from build123d import *

# Parameters (mm, degrees)
SKETCH1_W           = 669.925
SKETCH1_H           = 95.73895
BOSS_EXTRUDE1_DEPTH = 19.05
SKETCH2_R           = 12.7
CUT_EXTRUDE4_DEPTH  = 20.05


with BuildPart() as part:
    # Sketch1 → Boss-Extrude1 (new body)
    with BuildSketch(Plane(origin=(0, 0, 0), x_dir=(1, 0, 0), z_dir=(0, 1, 0))):
        with Locations((334.9625, 47.869475)):
            Rectangle(SKETCH1_W, SKETCH1_H)
    extrude(amount=BOSS_EXTRUDE1_DEPTH)

    # Sketch2 → Cut-Extrude4 (cut, through all)
    with BuildSketch(Plane.XZ):
        with Locations((334.9625, -82.78495)):
            Circle(SKETCH2_R)
    extrude(amount=-CUT_EXTRUDE4_DEPTH, mode=Mode.SUBTRACT)


solid = part.part
The listing builds one solid part. Answer for the finished solid, in the listing's coordinates (mm). Give positions to 0.01 mm unless a question says otherwise; leave off trailing zeros. Write each loop counter-clockwise with the first axis right and the second up, starting at its lowest first coordinate (ties: lowest second). Pieces come first, ordered by that corner, then holes.
1) For a pull along X with two mould halves and no side action, classify faces 1 (the face through (324.88, 9.39, -90.51)), 2 (the face through (0, 9, -47)), 3 (the face through (330, 9, -95.739)) as pulls with the +X half, pulls with the -X half, needs draft (parallel to the pull), parting line crosses it, or undercut.
2) Find the intervals of material crossed by L1, parallel to X at y = 11.5, z = -86.5 (3 decimals); L2, parallel to X at y = 8.5, z = -82 (3 decimals), in increasing order.
3) Section A-A (x = 335) is taken. Write down the section's boundary in (y, z) (3 decimals).
Response:
1. face 1: undercut
1. face 2: pulls with the -X half
1. face 3: needs draft
2. L1: x = 0 to 322.818, 347.107 to 669.925
2. L2: x = 0 to 322.287, 347.638 to 669.925
3. outline: (0, -95.739) - (19.05, -95.739) - (19.05, -95.485) - (0, -95.485) - close; (0, -70.085) - (19.05, -70.085) - (19.05, 0) - (0, 0) - close
